Autodesk Inventor part; units mm, degrees
ref_plane "YZ Plane" through (0, 0, 0) normal (1, 0, 0) x (0, 1, 0)
ref_plane "XZ Plane" through (0, 0, 0) normal (0, 1, 0) x (-1, 0, 0)
ref_plane "XY Plane" through (0, 0, 0) normal (0, 0, 1) x (1, 0, 0)
sketch "Boceto1" plane through (0, 0, 0) normal (0, 1, 0) x (-1, 0, 0)
  line L0 (-350, 400) -> (350, 400)
  line L1 (350, 400) -> (350, -400)
  line L2 (350, -400) -> (-350, -400)
  line L3 (-350, -400) -> (-350, 400)
  line L4 (-350, 400) -> (350, -400) construction
  line L5 (350, 400) -> (-350, -400) construction
  point P0 (0, 0)
  dimension "d0" = 700
  dimension "d1" = 800
extrude "Extrusión1" add sketch "Boceto1" along normal blind 150
fillet "Empalme1" radius 30 8 edges at (350, 150, 0) (0, 150, -400) (0, 150, 400) (-350, 150, 0) (-350, 75, 400) (350, 75, 400) (350, 75, -400) (-350, 75, -400)
sketch "Boceto2" plane through (0, 0, 0) normal (0, -1, 0) x (1, 0, 0)
  line L0 (-350, -370) -> (-350, 370)
  line L1 (-142.3817, -33.9222) -> (-350, -33.9222)
  line L2 (-350, -33.9222) -> (-350, 33.9222)
  line L3 (-350, 33.9222) -> (-142.3817, 33.9222)
  line L4 (-142.3817, 33.9222) -> (-142.3817, -33.9222)
  line L5 (-142.3817, -33.9222) -> (-350, 33.9222) construction
  line L6 (-350, -33.9222) -> (-142.3817, 33.9222) construction
  line L7 (0, 160.6517) -> (0, -134.4555)
  line L8 (142.3817, -33.9222) -> (350, -33.9222)
  line L9 (350, -33.9222) -> (350, 33.9222)
  line L10 (350, 33.9222) -> (142.3817, 33.9222)
  line L11 (142.3817, 33.9222) -> (142.3817, -33.9222)
  line L12 (142.3817, -33.9222) -> (350, 33.9222) construction
  line L13 (350, -33.9222) -> (142.3817, 33.9222) construction
  point P0 (0, 0)
  point P1 (-246.1908, 0)
  point P2 (246.1908, 0)
extrude "Extrusión2" add sketch "Boceto2" along normal blind 50
fillet "Empalme2" radius 30 4 edges at (-246.1908, -50, 33.9222) (-246.1908, -50, -33.9222) (246.1908, -50, 33.9222) (246.1908, -50, -33.9222)
sketch "Boceto3" plane through (-350, 0, 370) normal (-1, 0, 0) x (0, 0, 1)
  circle A0 centre (-370, -20) radius 10.25
  point P0 (-370, 0)
  dimension "d8" = 20.5
extrude "Extrusión3" add sketch "Boceto3" along normal blind 50
sketch "Boceto4" plane through (350, 0, -370) normal (1, 0, 0) x (0, 0, -1)
  circle A0 centre (-370, -20) radius 10.25
  circle A1 centre (-370, -20) radius 10.25
  point P0 (-370, 0)
extrude "Extrusión4" add sketch "Boceto4" along normal blind 50
sketch "Boceto5" plane through (0, 0, 0) normal (0, -1, 0) x (1, 0, 0)
  line L0 (-50, 325) -> (50, 325)
  line L1 (50, 325) -> (50, 225)
  line L2 (50, 225) -> (-50, 225)
  line L3 (-50, 225) -> (-50, 325)
  line L4 (-50, 325) -> (50, 225) construction
  line L5 (50, 325) -> (-50, 225) construction
  line L6 (-320, 400) -> (320, 400)
  line L7 (123.2582, 0) -> (-96.8001, 0)
  line L8 (-50, -325) -> (50, -325)
  line L9 (50, -325) -> (50, -225)
  line L10 (50, -225) -> (-50, -225)
  line L11 (-50, -225) -> (-50, -325)
  line L12 (-50, -325) -> (50, -225) construction
  line L13 (50, -325) -> (-50, -225) construction
  point P0 (0, 0)
  point P1 (0, 275)
  point P2 (0, -275)
  dimension "d13" = 100
  dimension "d14" = 100
  dimension "d15" = 75
extrude "Extrusión5" add sketch "Boceto5" along normal blind 21
properties part number "base_link"
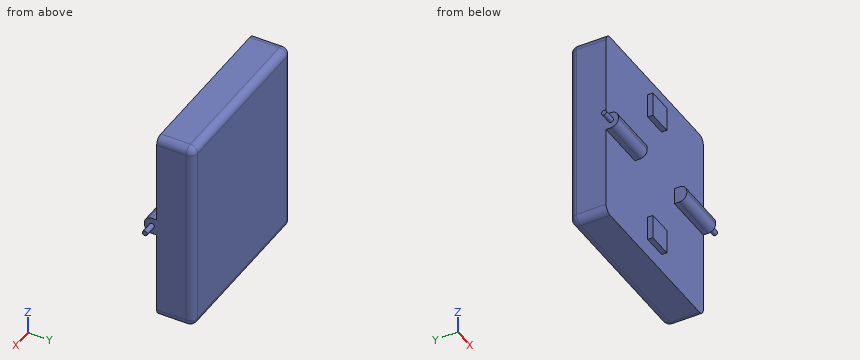
Read the model definition and answer for the solid it produces. Units are mm, in the model's axes. Coordinates: 2 decimals unless noted, no trailing zeros. Loops run counter-clockwise (first coordinate to the right, second up) from the corner with the lowest first, then second, coordinate; pieces in that order, holes last.
(1) The part is cut by section A-A (z = 308.5). Determine the outline of the cut face in (x, y).
Solution:
outline: (-350, 0) - (-50, 0) - (-50, -21) - (50, -21) - (50, 0) - (350, 0) - (350, 120) arc R30 ccw to (320, 150) - (-320, 150) arc R30 ccw to (-350, 120) - close
(2) The part is cut by section C-C (z = -161.5). Determine the outline of the cut face in (x, y), and give its area (3 significant figures).
Solution:
outline: (-350, 0) - (350, 0) - (350, 120) arc R30 ccw to (320, 150) - (-320, 150) arc R30 ccw to (-350, 120) - close
area: 105,000 mm2
(3) The part is cut by section B-B (x = -222). Determine the outline of the cut face in (y, z), and give its area (3 significant figures).
Solution:
outline: (-50, -3.92) arc R30 ccw to (-20, -33.92) - (0, -33.92) - (0, -400) - (120, -400) arc R30 ccw to (150, -370) - (150, 370) arc R30 ccw to (120, 400) - (0, 400) - (0, 33.92) - (-20, 33.92) arc R30 ccw to (-50, 3.92) - close
area: 123,000 mm2
(4) Consider line 1 along X through (y, z) = (21.5, -112.5); line 2 along Y through (x, z) = (238.5, 326); line 3 along Z through (x, y) = (-212.5, -4.5). Determine where each line is inside the solid, lowest interval first.
Solution:
line 1: x = -350 to 350
line 2: y = 0 to 150
line 3: z = -33.92 to 33.92
(5) Flat-ended cylindrical pins translate along their axes: pin 1 Ø6.5 at (y, z) = (-15.5, -295.5) entering from +X; pin 2 Ø8 at (x, z) = (15.5, 144.5) entering from -Y; pin 3 Ø16 at (x, y) = (-293.5, -9.5) entering from -Z. Find the tip coordinate at first contact, or state that the pin passes through.
Solution:
pin 1: stops at x = 50
pin 2: stops at y = 0
pin 3: stops at z = -33.92
